```python
from build123d import *

# Parameters (mm, degrees)
F3_R     = 9.525
F4_DEPTH = 304.801


with BuildPart() as f1:
    # F0 (on Right) → F1 (revolve)
    with BuildSketch(Plane.YZ):
        Polygon((0, 76.2), (0, 114.3), (-12.7, 114.3), (-12.7, 82.55), (-292.1, 82.55), (-292.1, 114.3), (-304.8, 114.3), (-304.8, 76.2), align=None)
    revolve(axis=Axis((0, 69.986956, 0), (0, 1, 0)))

    # F3 (on offset) → F4 (cut, through all)
    with BuildSketch(Plane.XZ.offset(304.8)):
        with Locations((0, 98.425)):
            Circle(F3_R)
        with Locations((-69.596985, 69.596985)):
            Circle(F3_R)
        with Locations((-98.425, 0)):
            Circle(F3_R)
        with Locations((-69.596985, -69.596985)):
            Circle(F3_R)
        with Locations((0, -98.425)):
            Circle(F3_R)
        with Locations((69.596985, -69.596985)):
            Circle(F3_R)
        with Locations((98.425, 0)):
            Circle(F3_R)
        with Locations((69.596985, 69.596985)):
            Circle(F3_R)
    extrude(amount=-F4_DEPTH, mode=Mode.SUBTRACT)


solid = f1.part
```
CAD build for the part. Positions are in the model's coordinates, mm. A direction names the side the tool comes from. Round coordinates to 2 decimals unless told otherwise and drop trailing zeros. Order: outer loops, then holes, each group sorted by start corner. A loop starts at its lowest first (then second) coordinate and runs counter-clockwise, first axis right, second up. Notation, with made-up numbers: (-27, 6.5) - (31, 6.5) arc R16 cw to (31, 28.5) - close; hole circle Ø9 at (68.25, 64.5). An arc over 180 degrees is marked (long way). Use CSV: the item, a comma, the result in double quotes. Start each with the question number.
1) Saw through at D-D (x = -52). List the corners of the cut face in (y, z), and give its area (3 significant figures).
2) Two-plate mould, pull along X, no slides. Class faces 1 (the cylindrical face through (60.08, -298.54, -69.18)), 2 (the flat face through (2, -304.8, -78)), 3 (the cylindrical face through (5.03, -298.54, -114.19)), 4 (the cylindrical face through (-89.34, -6.44, 2.86)): pulls with the +X half, pulls with the -X half, needs draft (parallel to the pull), parting line crosses it, or undercut.
3) Saw through at A-A (z = 0). Count the separate pieces of the cut face and the enclosed holes in it, and give its area (3 significant figures).
4) Saw through at C-C (z = 55). List the corners of the cut face in (x, y), and give its area (3 significant figures).
5) Wall check: L1, parallel to Y at x = 84.5, z = 57.5; L2, parallel to X at y = -286, z = -3.5; L3, parallel to Z at x = 40, y = -77. Give the ranges that are in metal, low to high. Write a range as [from, to].
6) Tool access for faces 5 (the flat face through (-76, -12.7, 33)), 6 (the cylindrical face through (-2.065, -298.539, -107.723)): list every direction of +Z, -Z, +X, -X, +Y, -Y with a clear straight run to the whole face (end or side of a thin tool).
7) Pin check, flat tips, straight feed: pin 1 Ø11.5 at (x, z) = (0, -98.425) entering from +Y; pin 2 Ø12 at (y, z) = (-54.5, -16) entering from -X; pin 3 Ø10 at (y, z) = (-198, 16) entering from +X; pin 4 Ø1.5 at (x, y) = (38.5, -126.5) entering from +Z. Stop position of each tip, or through.
Values follow:
1,outline,"(-304.8, -101.79) - (-292.1, -101.79) - (-292.1, -64.11) - (-12.7, -64.11) - (-12.7, -101.79) - (0, -101.79) - (0, -55.7) - (-304.8, -55.7) - close; (-304.8, 55.7) - (0, 55.7) - (0, 101.79) - (-12.7, 101.79) - (-12.7, 64.11) - (-292.1, 64.11) - (-292.1, 101.79) - (-304.8, 101.79) - close"
1,area,"7,040 mm2"
2,face 1,"undercut"
2,face 2,"needs draft"
2,face 3,"parting line crosses it"
2,face 4,"undercut"
3,separate pieces,"6"
3,enclosed holes,"0"
3,area,"4,520 mm2"
4,outline,"(-100.2, -304.8) - (-52.74, -304.8) - (-52.74, 0) - (-100.2, 0) - (-100.2, -12.7) - (-61.56, -12.7) - (-61.56, -292.1) - (-100.2, -292.1) - close; (52.74, -304.8) - (100.2, -304.8) - (100.2, -292.1) - (61.56, -292.1) - (61.56, -12.7) - (100.2, -12.7) - (100.2, 0) - (52.74, 0) - close"
4,area,"7,340 mm2"
5,L1,"y = [-304.8, -292.1], [-12.7, 0]"
5,L2,"x = [-82.48, -76.12], [76.12, 82.48]"
5,L3,"z = [-72.21, -64.86], [64.86, 72.21]"
6,face 5,"none"
6,face 6,"+Y, -Y"
7,pin 1,"passes through"
7,pin 2,"stops at x = -81.94"
7,pin 3,"stops at x = 81.81"
7,pin 4,"stops at z = 73.41"
